The listing builds one solid part. Answer for the finished solid, in the listing's coordinates (mm). Face numbers are marked on the shaded views. A direction names the side the tool comes from. Give positions to 0.01 mm unless a question says otherwise; leave off trailing zeros. Order: outer loops, then holes, each group sorted by start corner. A loop starts at its lowest first (then second) coordinate and runs counter-clockwise, first axis right, second up. Notation, with made-up numbers: (32, 86.25) -> (83, 86.25) arc R18 ccw to (83, 92.25) -> close; hole circle Ø2 at (-29, 81.5). An arc over 180 degrees is marked (long way). Answer as a JSON object with one key per item and string values. Group by question number.
```python
from build123d import *

# Parameters (mm, degrees)
F0_W     = 8
F0_H     = 30
F0_W_2   = 30
F0_H_2   = 8
F1_DEPTH = 224
F2_R     = 8
F3_R     = 8


with BuildPart() as f1:
    # F0 (on Front) → F1 (new body)
    with BuildSketch(Plane.XZ):
        with Locations((-20.8588695079, 39.1709680259)):
            Rectangle(F0_W, F0_H)
        Polygon((-16.8588695079, 24.1709680259), (-24.8588695079, 24.1709680259), (-24.8588695079, 20.1709680259), align=None)
        Polygon((28.1411304921, -20.8290319741), (-16.8588695079, 24.1709680259), (-24.8588695079, 20.1709680259), (24.1411304921, -28.8290319741), align=None)
        with Locations((43.1411304921, -24.8290319741)):
            Rectangle(F0_W_2, F0_H_2)
        Polygon((28.1411304921, -28.8290319741), (28.1411304921, -20.8290319741), (24.1411304921, -28.8290319741), align=None)
    extrude(amount=F1_DEPTH)

    # F2
    f2_edges = [f1.edges().sort_by_distance(p)[0] for p in [
        (-16.85887, -112, 24.170968),
        (28.14113, -112, -20.829032),
    ]]
    fillet(f2_edges, radius=F2_R)

    # F3
    f3_edges = [f1.edges().sort_by_distance(p)[0] for p in [
        (-24.85887, -112, 20.170968),
        (24.14113, -112, -28.829032),
    ]]
    fillet(f3_edges, radius=F3_R)


solid = f1.part
```
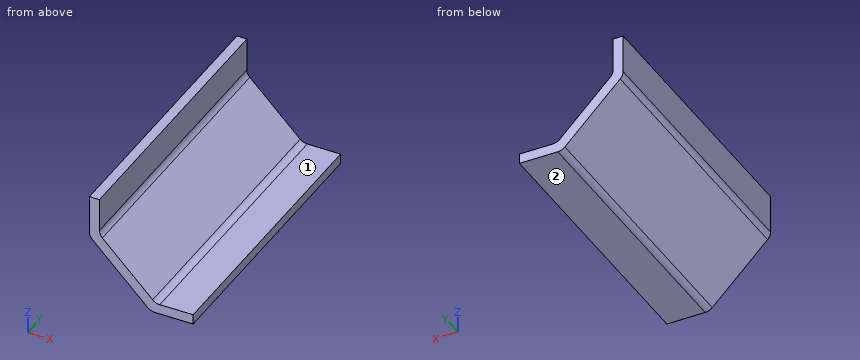
(1) A cutting plane is placed at C-C (x = 42.5). Determine the outline of the cut face in (y, z), and give its area (3 significant figures).
(2) A cutting plane is placed at B-B (z = 42). Determine the outline of the cut face in (x, y), and give its area (3 significant figures).
(3) Flat-ended cylindrical pins translate along their axes: pin 1 Ø12 at (x, z) = (-8, 41) entering from -Y (1 decimal); pin 2 Ø12 at (x, y) = (38, -183) entering from +Z; pin 3 Ø13.5 at (y, z) = (-57.5, 38.5) entering from +X; pin 4 Ø6 at (y, z) = (-189, -7.5) entering from +X. Find the tip coordinate at first contact, or state that the pin passes through.
(4) Find the intervals of material crossed by line 1 along X through (y, z) = (-169, 51.5); line 2 along Z through (x, y) = (36, -34); line 3 along X through (y, z) = (-185, -22.5), in increasing order. Write a range as [from, to].
(5) A cutting plane is placed at A-A (y = -193). Determine the outline of the cut face in (x, z), and give its area (3 significant figures).
(6) Which of the six approach directions +Z, -Z, +X, -X, +Y, -Y give full straight-line access (tool end or side, diameter ignored) to the marked faces 1 and 2?
Check sheet entries:
{
 "1": {"outline": "(-224, -28.83) -> (0, -28.83) -> (0, -20.83) -> (-224, -20.83) -> close", "area": "1,790 mm2"},
 "2": {"outline": "(-24.86, -224) -> (-16.86, -224) -> (-16.86, 0) -> (-24.86, 0) -> close", "area": "1,790 mm2"},
 "3": {"pin 1": "passes through", "pin 2": "stops at z = -20.83", "pin 3": "stops at x = -16.86", "pin 4": "stops at x = 17.81"},
 "4": {"line 1": "x = [-24.86, -16.86]", "line 2": "z = [-28.83, -20.83]", "line 3": "x = [17.81, 58.14]"},
 "5": {"outline": "(-24.86, 23.48) arc R8 ccw to (-22.52, 17.83) -> (21.8, -26.49) arc R8 ccw to (27.45, -28.83) -> (58.14, -28.83) -> (58.14, -20.83) -> (31.45, -20.83) arc R8 cw to (25.8, -18.49) -> (-14.52, 21.83) arc R8 cw to (-16.86, 27.48) -> (-16.86, 54.17) -> (-24.86, 54.17) -> close", "area": "1,080 mm2"},
 "6": {"face 1": "+Z, +X, +Y, -Y", "face 2": "-Z, +X, -X, +Y, -Y"}
}
